```python
from build123d import *

# Parameters (mm, degrees)
SKETCH1_W           = 20
SKETCH1_H           = 30
BOSS_EXTRUDE1_DEPTH = 5
SKETCH2_R           = 1.75
CUT_EXTRUDE1_DEPTH  = 8
SKETCH3_R           = 1.75
CUT_EXTRUDE2_DEPTH  = 37.400549446
SKETCH4_W           = 6
SKETCH4_H           = 3
CUT_EXTRUDE3_DEPTH  = 9


with BuildPart() as part:
    # Sketch1 → Boss-Extrude1 (new body)
    with BuildSketch(Plane(origin=(0, 0, 0), x_dir=(1, 0, 0), z_dir=(0, 1, 0))):
        with Locations((10, 15)):
            Rectangle(SKETCH1_W, SKETCH1_H)
    extrude(amount=BOSS_EXTRUDE1_DEPTH)

    # Sketch2 → Cut-Extrude1 (cut)
    with BuildSketch(Plane(origin=(0, 5, 0), x_dir=(1, 0, 0), z_dir=(0, 1, 0))):
        with Locations(Location((5.5, 15, 0), (0, 0, 270))):
            Circle(SKETCH2_R)
    extrude(amount=-CUT_EXTRUDE1_DEPTH, mode=Mode.SUBTRACT)

    # Sketch3 → Cut-Extrude2 (cut, through all)
    with BuildSketch(Plane(origin=(0, 5, 0), x_dir=(1, 0, 0), z_dir=(0, 1, 0))):
        with Locations(Location((10, 25, 0), (0, 0, 270))):
            Circle(SKETCH3_R)
        with Locations(Location((10, 5, 0), (0, 0, 270))):
            Circle(SKETCH3_R)
    extrude(amount=-CUT_EXTRUDE2_DEPTH, mode=Mode.SUBTRACT)

    # Sketch4 → Cut-Extrude3 (cut)
    with BuildSketch(Plane.ZY):
        with Locations((-15, 1.5)):
            Rectangle(SKETCH4_W, SKETCH4_H)
    extrude(amount=-CUT_EXTRUDE3_DEPTH, mode=Mode.SUBTRACT)


solid = part.part
```
Check sheet for the modelled part. Datum: model origin and axes. Units: mm. A direction names the side the tool comes from. Round coordinates to 2 decimals unless told otherwise and drop trailing zeros. Order: outer loops, then holes, each group sorted by start corner. A loop starts at its lowest first (then second) coordinate and runs counter-clockwise, first axis right, second up.
1) Section check D-D (z = -15). Record the boundary of the cut face in (x, y).
2) Scan lines: line 1 (X direction, y = 3.95, z = -25); line 2 (Z direction, x = 11, y = 2.8); line 3 (Z direction, x = 4.5, y = 2.75). Record each from-to range of solid material in increasing order.
3) Mould release check, pull along X, two halves, no side actions. Record for faces 3 (the flat face through (10, 2, -30)), 4 (the flat face through (20, 2, -15)), 5 (the cylindrical face through (3.95, 4.01, -14.19)), 6 (the cylindrical face through (10.08, 2.54, -26.75)): +X half, -X half, draft (parallel to the pull), parting line (faces both ways), or undercut.
4) Section check A-A (z = -5). Record the boundary of the cut face in (x, y).
5) Section check B-B (y = 1.15). Record the boundary of the cut face in (x, z), and give its area (3 significant figures).
6) Tool access check on faces 1 (the flat face through (3, 3, -15)), 2 (the flat face through (0, 4, -15)). Record the directions out of +Z, -Z, +X, -X, +Y, -Y that give a thin tool (end or side, any length) a straight path to the whole face; none if there is none.
7) Go/stop test with flat-tipped pins: pin 1 Ø2.5 at (y, z) = (1.5, -14.5) entering from -X; pin 2 Ø3 at (x, z) = (10, -5) entering from +Y. Record where each tip stops, or that it passes through.
8) Section check C-C (x = 5.5). Record the boundary of the cut face in (y, z), and give its area (3 significant figures).
Result:
1. outline: (0, 3) - (3.75, 3) - (3.75, 5) - (0, 5) - close; (7.25, 3) - (9, 3) - (9, 0) - (20, 0) - (20, 5) - (7.25, 5) - close
2. line 1: x = 0 to 8.25, 11.75 to 20
2. line 2: z = -30 to -26.44, -23.56 to -6.44, -3.56 to 0
2. line 3: z = -30 to -18, -12 to 0
3. face 3: draft
3. face 4: +X half
3. face 5: undercut
3. face 6: undercut
4. outline: (0, 0) - (8.25, 0) - (8.25, 5) - (0, 5) - close; (11.75, 0) - (20, 0) - (20, 5) - (11.75, 5) - close
5. outline: (0, -30) - (20, -30) - (20, 0) - (0, 0) - (0, -12) - (9, -12) - (9, -18) - (0, -18) - close; hole circle Ø3.5 at (10, -25); hole circle Ø3.5 at (10, -5)
5. area: 527 mm2
6. face 1: -X, -Y
6. face 2: +Z, -Z, -X, +Y, -Y
7. pin 1: stops at x = 9
7. pin 2: passes through
8. outline: (0, -30) - (5, -30) - (5, -16.75) - (3, -16.75) - (3, -18) - (0, -18) - close; (0, -12) - (3, -12) - (3, -13.25) - (5, -13.25) - (5, 0) - (0, 0) - close
8. area: 125 mm2
